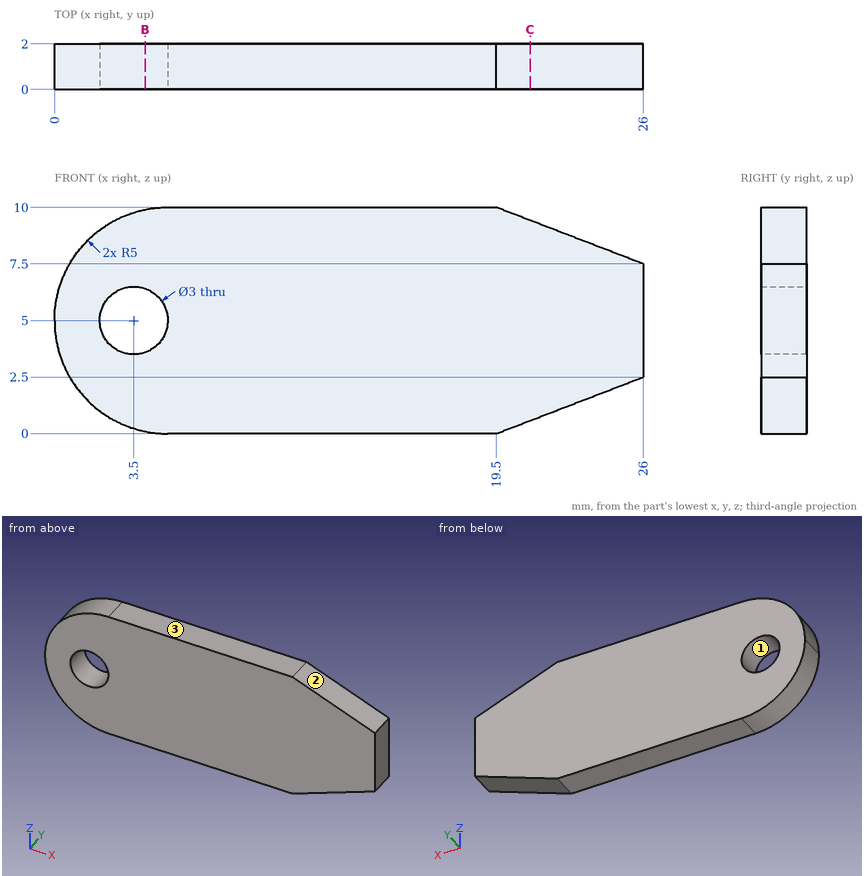
The figure shows three views and two pictorial views of one solid part (mm, origin at its lowest corner). Answer the questions. Round coordinates to 2 decimals unless told otherwise and drop trailing zeros. Write each loop counter-clockwise with the first axis right and the second up, starting at its lowest first coordinate (ties: lowest second). Pieces come first, ordered by that corner, then holes. Notation, with made-up numbers: (17.25, 3.25) - (42.25, 3.25) arc R11 ccw to (42.25, 24.25) - close; hole circle Ø1 at (33.5, 29.25). An arc over 180 degrees is marked (long way). Use one line per item in the form item = value. Start each with the question number.
Item 1: A cutting plane is placed at C-C (x = 21). Write down the section's boundary in (y, z), plus the area to 3 significant figures.
Item 2: A flat-ended cylindrical pin translates along its axis: pin 1 Ø6 at (x, z) = (8, 6) entering from -Y. Find the tip coordinate at first contact, or state that the pin passes through.
Item 3: Find the intervals of material crossed by line 1 (X direction, y = 1.35, z = 5); line 2 (X direction, y = 1.7, z = 4); line 3 (Z direction, x = 2.5, y = 1.7), in increasing order. Write a range as [from, to].
Item 4: Determine the mould class of the marked faces 1, 2 and 3 for opening direction X: +X half, -X half, draft (parallel to the pull), parting line (faces both ways), or undercut.
Item 5: A cutting plane is placed at B-B (x = 4). Write down the section's boundary in (y, z).
The answers:
q1.outline = (0, 0.58) - (2, 0.58) - (2, 9.42) - (0, 9.42) - close
q1.area = 17.7 mm^2
q2.pin_1 = 0
q3.line_1 = [0, 2], [5, 26]
q3.line_2 = [0.1, 2.38], [4.62, 26]
q3.line_3 = [0.67, 3.88], [6.12, 9.33]
q4.face_1 = undercut
q4.face_2 = +X half
q4.face_3 = draft
q5.outline = (0, 0.1) - (2, 0.1) - (2, 3.59) - (0, 3.59) - close; (0, 6.41) - (2, 6.41) - (2, 9.9) - (0, 9.9) - close
